from build123d import *

# Parameters (mm, degrees)
BOSS_EXTRUDE1_DEPTH = 3
SKETCH2_R           = 1.06
CUT_EXTRUDE1_DEPTH  = 3


with BuildPart() as part:
    # Model → Boss-Extrude1 (new body)
    with BuildSketch(Plane.XY):
        Polygon((85.038482334, 125.842661122), (85.641402334, 125.931201122), (85.995047634, 125.896821579), (86.992422179, 125.445319522), (86.992422179, 124.852599522), (85.995047634, 124.401097464), (85.641402334, 124.366717921), (85.038482334, 124.455257921), (84.752432117, 123.387727108), (85.31884426, 123.162940226), (85.607924576, 122.95635), (86.245924576, 122.06665), (85.949564326, 121.553339567), (84.86006114, 121.661009882), (84.536608908, 121.80806635), (84.058733602, 122.186202635), (83.277245674, 121.404714707), (83.65538196, 120.926839402), (83.802438428, 120.60338717), (83.910108743, 119.513883983), (83.39679831, 119.217523733), (82.50709831, 119.855523733), (82.300508083, 120.14460405), (82.075721201, 120.711016193), (81.008190388, 120.424965975), (81.096730388, 119.822045975), (81.062350845, 119.468400675), (80.610848788, 118.471026131), (80.018128788, 118.471026131), (79.566626731, 119.468400675), (79.532247188, 119.822045975), (79.620787188, 120.424965975), (78.553256375, 120.711016193), (78.328469493, 120.14460405), (78.121879267, 119.855523733), (77.232179267, 119.217523733), (76.718868834, 119.513883983), (76.826539148, 120.60338717), (76.973595617, 120.926839402), (77.351731902, 121.404714707), (76.570243974, 122.186202635), (76.092368668, 121.80806635), (75.768916436, 121.661009882), (74.67941325, 121.553339567), (74.383053, 122.06665), (75.021053, 122.95635), (75.310133317, 123.162940226), (75.87654546, 123.387727108), (75.590503, 124.45526), (74.987583, 124.36672), (74.633937545, 124.401097943), (73.636563, 124.8526), (73.636563, 125.44532), (74.633937545, 125.896822057), (74.987582844, 125.9312016), (75.590502844, 125.8426616), (75.876553062, 126.910192413), (75.310140919, 127.134979295), (75.021060603, 127.341569522), (74.383060603, 128.231269522), (74.679420853, 128.744579955), (75.768924039, 128.63690964), (76.092376271, 128.489853171), (76.570251576, 128.111716886), (77.351739505, 128.893204814), (76.973603219, 129.37108012), (76.826546751, 129.694532352), (76.718876436, 130.784035538), (77.232186869, 131.080395788), (78.121886869, 130.442395788), (78.328477095, 130.153315471), (78.553263977, 129.586903328), (79.62079479, 129.872953546), (79.53225479, 130.475873546), (79.566634333, 130.829518846), (80.018136391, 131.826893391), (80.610856391, 131.826893391), (81.062358448, 130.829518846), (81.096737991, 130.475873546), (81.008197991, 129.872953546), (82.075728804, 129.586903328), (82.300515686, 130.153315471), (82.507105912, 130.442395788), (83.396805912, 131.080395788), (83.910116345, 130.784035538), (83.80244603, 129.694532352), (83.655389562, 129.37108012), (83.277253277, 128.893204814), (84.058741205, 128.111716886), (84.536616511, 128.489853171), (84.860068742, 128.63690964), (85.949571929, 128.744579955), (86.245932179, 128.231269522), (85.607932179, 127.341569522), (85.318851862, 127.134979295), (84.75243916, 126.910193822), align=None)
    extrude(amount=BOSS_EXTRUDE1_DEPTH)

    # Sketch2 → Cut-Extrude1 (cut)
    with BuildSketch(Plane.XY.offset(3)):
        with Locations((80.314492489, 125.148960513)):
            Circle(SKETCH2_R)
    extrude(amount=-CUT_EXTRUDE1_DEPTH, mode=Mode.SUBTRACT)


solid = part.part
Work out the finished part from the listing and answer in its coordinate system (mm). A direction names the side the tool comes from. Give positions to 0.01 mm unless a question says otherwise; leave off trailing zeros. Loops run counter-clockwise (first coordinate to the right, second up) from the corner with the lowest first, then second, coordinate; pieces in that order, holes last. Notation, with made-up numbers: (-5.5, 56) -> (18.5, 56) arc R32 cw to (18.5, 92) -> close; hole circle Ø2 at (-17.5, 88). An arc over 180 degrees is marked (long way). Use a Markdown table: item, result. Add a question column.
1) Consider line 1 along X through (y, z) = (120, 2.15); line 2 along Y through (x, z) = (75.5, 1.25); line 3 along X through (y, z) = (119.75, 0.2). Determine where each line is inside the solid, lowest interval first.
2) This flat-tipped pin is pushed along its axis until it touches: P1, Ø1.5, axis at y = 120.5, z = 1.5, coming from the -X side. Where does it stop, or does it pass through?
3) Which of the six approach directions +Z, -Z, +X, -X, +Y, -Y give full straight-line access (tool end or side, diameter ignored) to faces 4 (the flat face through (86.5, 124.63, 1.48)), 5 (the flat face through (75.232, 121.608, 1.479)), 6 (the flat face through (77.671, 130.766, 1.479))?
4) The part is cut by section A-A, the plane y = 123.75. Determine the outline of the cut face in (x, z), plus the area to 3 significant figures.
5) For a pull along X with two mould halves and no side action, classify faces 1 (the flat face through (74.13, 125.67, 1.48)), 2 (the flat face through (83.857, 130.247, 1.479)), 3 (the flat face through (85.412, 121.606, 1.479)) as +X half, -X half, draft (parallel to the pull), parting line (faces both ways), or undercut.
Reported:
| question | item | result |
|---|---|---|
| 1 | line 1 | x = 76.77 to 78.23, 79.56 to 81.07, 82.4 to 83.86 |
| 1 | line 2 | y = 121.63 to 123.24, 124.44 to 125.86, 127.06 to 128.66 |
| 1 | line 3 | x = 76.74 to 77.97, 79.54 to 81.09, 82.65 to 83.89 |
| 2 | P1 | stops at x = 76.74 |
| 3 | face 4 | +Z, -Z, +X |
| 3 | face 5 | +Z, -Z, -Y |
| 3 | face 6 | +Z, -Z, +Y |
| 4 | outline | (75.78, 0) -> (84.85, 0) -> (84.85, 3) -> (75.78, 3) -> close |
| 4 | area | 27.2 mm^2 |
| 5 | face 1 | -X half |
| 5 | face 2 | +X half |
| 5 | face 3 | undercut |
